Job drawing, mm, ordinate dimensions from the low corner. One solid piece. Give positions to 0.01 mm unless a question says otherwise; leave off trailing zeros. Write each loop counter-clockwise with the first axis right and the second up, starting at its lowest first coordinate (ties: lowest second). Pieces come first, ordered by that corner, then holes. Notation, with made-up numbers: M 41,36.25 L 45,36.25 A17 cw 45,64.25 Z; hole C 43,51.5 d11. An arc over 180 degrees is marked long. Answer as CSV lines item,"result". Start each with the question number.
1) Pin check, flat tips, straight feed: pin 1 Ø1.6 at (y, z) = (36, 1) entering from -X; pin 2 Ø1.5 at (x, z) = (34, 3.5) entering from +Y; pin 3 Ø1 at (x, z) = (37, 1) entering from +Y. Stop position of each tip, or through.
2) Slice it at C-C, the plane z = 2.8. Give the cut face in (x, y).
3) Slice it at A-A, the plane y = 40. Give the cut face in (x, z), plus the area to 3 significant figures.
4) Wall check: line 1 along Y through (x, z) = (50.5, 1.4); line 2 along X through (y, z) = (40, 1.4); line 3 along Y through (x, z) = (50.5, 3.3). Give the ranges that are in metal, low to high. Write a range as from..to.
5) Slice it at D-D, the plane x = 29.5. Give the cut face in (y, z).
6) Slice it at B-B, the plane x = 40. Give the cut face in (y, z), plus the area to 3 significant figures.
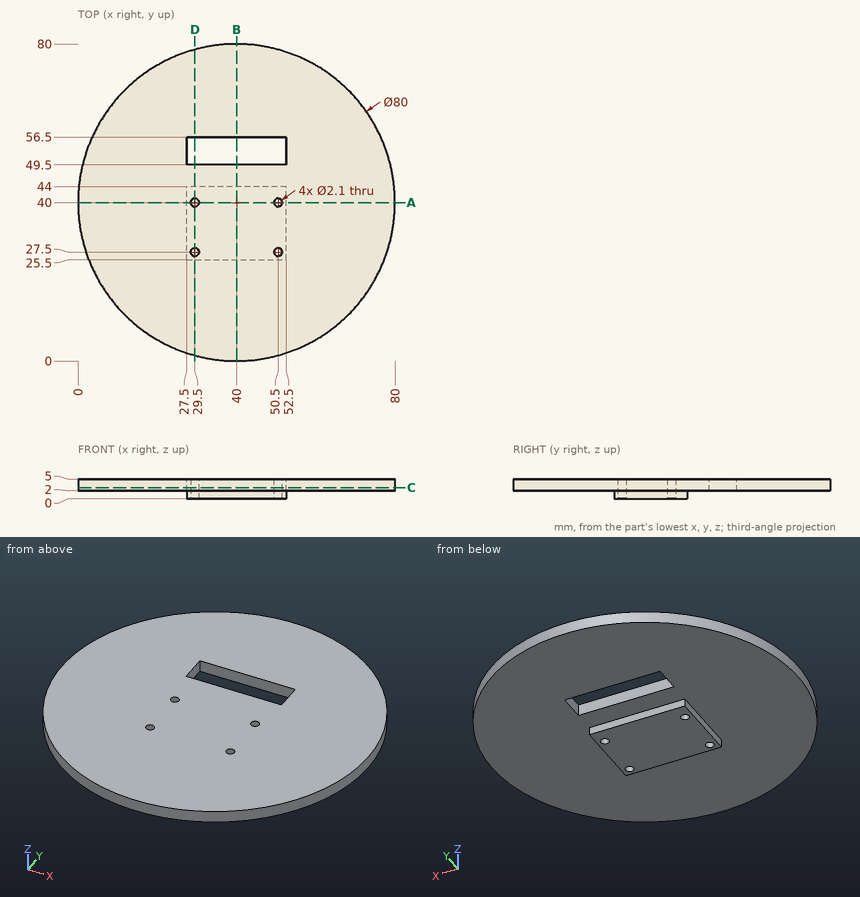
Found:
1,pin 1,"x = 27.5"
1,pin 2,"y = 79.65"
1,pin 3,"y = 44"
2,outline,"C 40,40 d80; hole M 27.5,49.5 L 52.5,49.5 L 52.5,56.5 L 27.5,56.5 Z; hole C 29.5,27.5 d2.1; hole C 29.5,40 d2.1; hole C 50.5,27.5 d2.1; hole C 50.5,40 d2.1"
3,outline,"M 0,2 L 27.5,2 L 27.5,0 L 28.45,0 L 28.45,5 L 0,5 Z; M 30.55,0 L 49.45,0 L 49.45,5 L 30.55,5 Z; M 51.55,0 L 52.5,0 L 52.5,2 L 80,2 L 80,5 L 51.55,5 Z"
3,area,"269 mm²"
4,line 1,"25.5..26.45, 28.55..38.95, 41.05..44"
4,line 2,"27.5..28.45, 30.55..49.45, 51.55..52.5"
4,line 3,"1.4..26.45, 28.55..38.95, 41.05..49.5, 56.5..78.6"
5,outline,"M 1.4,2 L 25.5,2 L 25.5,0 L 26.45,0 L 26.45,5 L 1.4,5 Z; M 28.55,0 L 38.95,0 L 38.95,5 L 28.55,5 Z; M 41.05,0 L 44,0 L 44,2 L 49.5,2 L 49.5,5 L 41.05,5 Z; M 56.5,2 L 78.6,2 L 78.6,5 L 56.5,5 Z"
6,outline,"M 0,2 L 25.5,2 L 25.5,0 L 44,0 L 44,2 L 49.5,2 L 49.5,5 L 0,5 Z; M 56.5,2 L 80,2 L 80,5 L 56.5,5 Z"
6,area,"256 mm²"
